Verification items for this drawing (mm, ordinates from the low corner). A direction names the side the tool comes from. Give positions to 0.01 mm unless a question says otherwise; leave off trailing zeros. Loops run counter-clockwise (first coordinate to the right, second up) from the corner with the lowest first, then second, coordinate; pieces in that order, holes last. Notation, with made-up numbers: M 30,66 L 70,66 A18 cw 70,96 Z; hole C 76,18 d9. An arc over 180 degrees is marked long. Use one line per item in the form item = value.
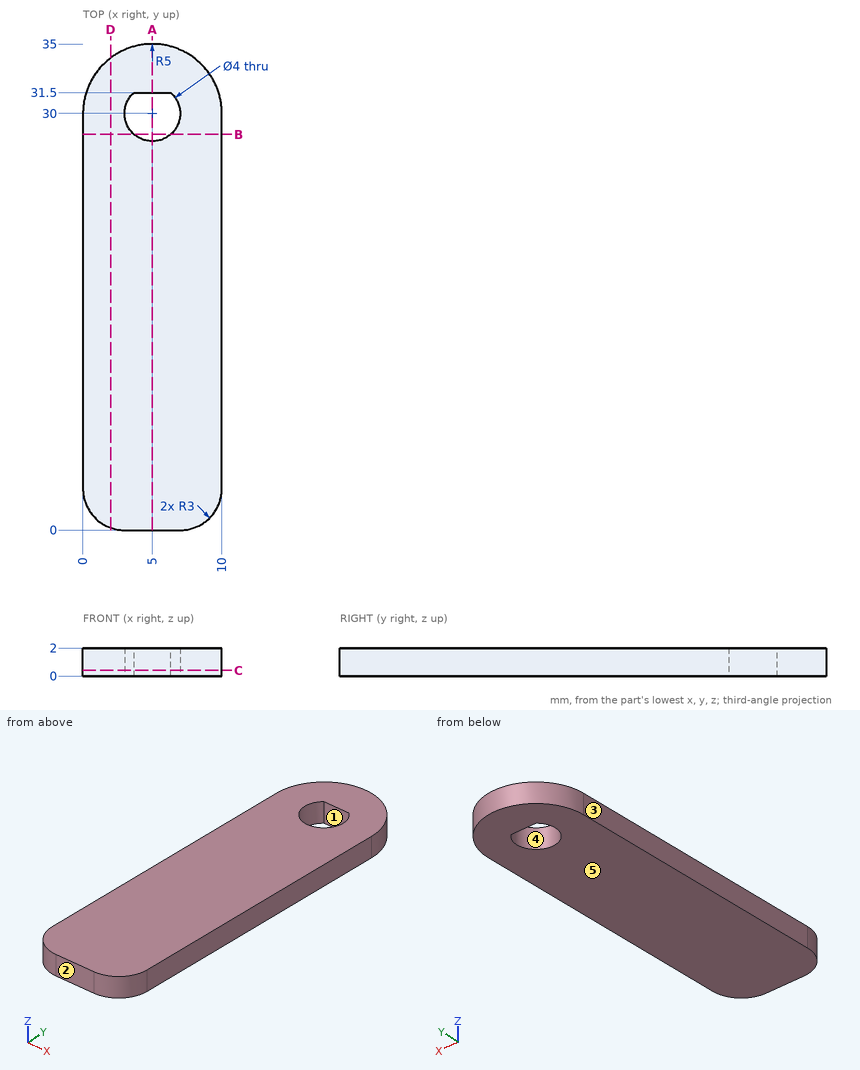
1) Scan lines: line 1 (X direction, y = 30, z = 1.6); line 2 (Y direction, x = 3.5, z = 0.4); line 3 (Y direction, x = 1, z = 0.2). Record each from-to range of solid material in increasing order.
Evaluation:
line_1 = 0 to 3, 7 to 10
line_2 = 0 to 28.68, 31.32 to 34.77
line_3 = 0.76 to 33
2) Section check B-B (y = 28.5). Record the cut outline in (x, z), then the cut area to 3 significant figures.
Evaluation:
outline = M 0,0 L 3.68,0 L 3.68,2 L 0,2 Z; M 6.32,0 L 10,0 L 10,2 L 6.32,2 Z
area = 14.7 mm^2
3) Depth check by flat-ended pin: pin 1 Ø6 at (x, y) = (3, 20.5) entering from -Z. Enter the tip coordinate at first touch or a pass-through.
Evaluation:
pin_1 = 0
4) Release check for a two-part mould opening along X. For the marked faces 3, 4 and 5 record: pulls with the +X half, pulls with the -X half, needs draft (parallel to the pull), parting line crosses it, or undercut.
Evaluation:
face_3 = pulls with the -X half
face_4 = undercut
face_5 = needs draft
5) Section check A-A (x = 5). Record the cut outline in (y, z).
Evaluation:
outline = M 0,0 L 28,0 L 28,2 L 0,2 Z; M 31.5,0 L 35,0 L 35,2 L 31.5,2 Z
6) Set-up check for the marked faces 1 and 2: record each of +Z, -Z, +X, -X, +Y, -Y from which the full face is reachable in a straight line by a thin tool's end or side.
Evaluation:
face_1 = +Z, -Z
face_2 = +Z, -Z, +X, -X, -Y
7) Section check C-C (z = 0.4). Record the cut outline in (x, y), then the cut area to 3 significant figures.
Evaluation:
outline = M 0,3 A3 ccw 3,0 L 7,0 A3 ccw 10,3 L 10,30 A5 ccw 0,30 Z; hole M 3.68,31.5 A2 ccw long 6.32,31.5 Z
area = 324 mm^2
8) Section check D-D (x = 2). Record the cut outline in (y, z).
Evaluation:
outline = M 0.17,0 L 34,0 L 34,2 L 0.17,2 Z
